Autodesk Inventor part; units mm, degrees
ref_plane "YZ Plane" through (0, 0, 0) normal (1, 0, 0) x (0, 1, 0)
ref_plane "XZ Plane" through (0, 0, 0) normal (0, 1, 0) x (-1, 0, 0)
ref_plane "XY Plane" through (0, 0, 0) normal (0, 0, 1) x (1, 0, 0)
sketch "Sketch1" plane through (0, 0, 0) normal (0, 1, 0) x (-1, 0, 0)
  line L0 (-21, -21) -> (21, -21)
  line L1 (21, -21) -> (21, 21)
  line L2 (21, 21) -> (-21, 21)
  line L3 (-21, 21) -> (-21, -21)
  line L4 (-21, -21) -> (21, 21) construction
  line L5 (21, -21) -> (-21, 21) construction
  point P0 (0, 0)
  dimension "d0" = 42
extrude "Extrusion1" add sketch "Sketch1" along normal blind 5
sketch "Sketch2" plane through (0, 0, 0) normal (0, 1, 0) x (1, 0, 0)
  circle A0 centre (0, 0) radius 21
  dimension "d3" = 42
extrude "Extrusion2" add sketch "Sketch2" along normal blind 51
sketch "Sketch3" plane through (0, 51, 0) normal (0, 1, 0) x (1, 0, 0)
  circle A0 centre (0, 0) radius 12.5
  dimension "d6" = 25
extrude "Extrusion3" add sketch "Sketch3" along normal blind 2
sketch "Sketch4" plane through (0, 51, 0) normal (0, 1, 0) x (1, 0, 0)
  circle A0 centre (0, 0) radius 4
  dimension "d9" = 8
extrude "Extrusion4" add sketch "Sketch4" along normal blind 22
sketch "Sketch5" plane through (0, 51, 0) normal (0, 1, 0) x (1, 0, 0)
  line L0 (-12.3744, -12.3744) -> (12.3744, -12.3744)
  line L1 (12.3744, -12.3744) -> (12.3744, 12.3744)
  line L2 (12.3744, 12.3744) -> (-12.3744, 12.3744)
  line L3 (-12.3744, 12.3744) -> (-12.3744, -12.3744)
  line L4 (-12.3744, -12.3744) -> (12.3744, 12.3744) construction
  line L5 (12.3744, -12.3744) -> (-12.3744, 12.3744) construction
  point P0 (0, 0)
  dimension "d15" = 35
hole "Hole1" at (12.3744, 51, -12.3744) at (-12.3744, 51, -12.3744) at (-12.3744, 51, 12.3744) at (12.3744, 51, 12.3744) direction (0, -1, 0) diameter 3.242 depth 6 tip angle 118
sketch "Sketch6" plane through (0, 73, 0) normal (0, 1, 0) x (1, 0, 0)
  point P0 (0, 0)
  point P1 (0, 0)
hole "Hole2" at (0, 73, 0) direction (0, -1, 0) diameter 2.459 depth 6 tip angle 118
chamfer "Chamfer1" distance 3 angle 45 4 edges at (21, 2.5, -21) (-21, 2.5, -21) (21, 2.5, 21) (-21, 2.5, 21)
sketch "Sketch7" plane through (0, 0, 0) normal (0, 1, 0) x (-1, 0, 0)
  circle A0 centre (0, 0) radius 11
  dimension "d30" = 22
extrude "Extrusion5" cut sketch "Sketch7" along normal blind 2
sketch "Sketch8" plane through (0, 0, 0) normal (0, 1, 0) x (-1, 0, 0)
  line L0 (15.5, 15.5) -> (-15.5, 15.5)
  line L1 (-15.5, 15.5) -> (-15.5, -15.5)
  line L2 (-15.5, -15.5) -> (15.5, -15.5)
  line L3 (15.5, -15.5) -> (15.5, 15.5)
  line L4 (15.5, 15.5) -> (-15.5, -15.5) construction
  line L5 (-15.5, 15.5) -> (15.5, -15.5) construction
  point P0 (0, 0)
  dimension "d33" = 31
hole "Hole3" at (15.5, 0, 15.5) at (-15.5, 0, 15.5) at (-15.5, 0, -15.5) at (15.5, 0, -15.5) direction (0, 1, 0) diameter 3.7 depth 5
sketch "Sketch9" plane through (0, 5, 0) normal (0, 1, 0) x (1, 0, 0)
  arc A0 (-15.9176, -13.6978) -> (-13.6978, -15.9176) centre (-15.5, -15.5) ccw
  circle A1 centre (-15.5, 15.5) radius 1.85
  arc A2 (15.9176, 13.6978) -> (13.6978, 15.9176) centre (15.5, 15.5) ccw
  circle A3 centre (15.5, -15.5) radius 1.85
  point P0 (0, 0)
hole "Hole4" at (-15.5, 5, 15.5) at (-15.5, 5, -15.5) at (15.5, 5, -15.5) at (15.5, 5, 15.5) direction (0, -1, 0) diameter 6.6 depth 3 tip angle 118
properties part number "911-42-reducer-long"
Work out the finished part from the listing and answer in its coordinate system (mm). A direction names the side the tool comes from. Coordinates: 2 decimals unless noted, no trailing zeros. Order: outer loops, then holes, each group sorted by start corner. A loop starts at its lowest first (then second) coordinate and runs counter-clockwise, first axis right, second up. Notation, with made-up numbers: (-14, 79.5) - (29, 79.5) arc R19 ccw to (29, 95.5) - close; hole circle Ø1 at (-29.5, 37). An arc over 180 degrees is marked (long way). Put each result on its own line as item: value. Start each with the question number.
1) Find section D-D (y = 34.5). Give the vertices of the cut face in (x, z).
2) Find section C-C (x = 6). Give the vertices of the cut face in (y, z), plus the area to 3 significant figures.
3) Find section B-B (z = -15.5). Give the vertices of the cut face in (x, y).
4) For faces 4 (the cylindrical face through (10.767, 47.958, 12.163)), 5 (the cylindrical face through (15.4, 3.5, -18.8)), 6 (the cylindrical face through (2.38, 0.99, 10.74)), 7 (the flat face through (18, 5, 18)), determine the directions among +Z, -Z, +X, -X, +Y, -Y from which every point of the face is accessible in a straight line to the end or side of a thin tool.
5) Find the intervals of material crossed by line 1 (Z direction, x = -15.5, y = 0.45); line 2 (X direction, y = 3, z = -15), in increasing order. Write a range as from..to.
6) For a pull along Y with two mould halves and no side action, classify faces 1 (the flat face through (-3, 53, -3)), 2 (the flat face through (-14, 5, -14)), 3 (the cylindrical face through (-10.792, 47.958, 12.023)) as released by +Y, released by -Y, zero draft, split by the parting line, or undercut.
7) Flat-ended cylindrical pins translate along their axes: pin 1 (3 mm diameter, centred on y = 9.5, z = 13, fed in from +X); pin 2 (1 mm diameter, centred on x = 2.5, y = 9, fed in from +Z); pin 3 (2.5 mm diameter, centred on x = 15, z = -15.5, fed in from -Y). Find the tip coordinate at first contact, or state that the pin passes through.
8) Find section A-A (x = -15.5). Give the vertices of the cut face in (y, z).
Results list:
1. outline: circle Ø42 at (0, 0)
2. outline: (0, -21) - (5, -21) - (5, -20.12) - (51, -20.12) - (51, -10.97) - (53, -10.97) - (53, 10.97) - (51, 10.97) - (51, 20.12) - (5, 20.12) - (5, 21) - (0, 21) - (0, 9.22) - (2, 9.22) - (2, -9.22) - (0, -9.22) - close
2. area: 2,070 mm^2
3. outline: (-21, 0) - (-17.35, 0) - (-17.35, 1.13) - (-18.8, 2) - (-18.8, 5) - (-21, 5) - close; (-14.17, 5) - (-12.2, 5) - (-12.2, 2) - (-13.65, 1.13) - (-13.65, 0) - (13.65, 0) - (13.65, 1.13) - (12.2, 2) - (12.2, 5) - (14.17, 5) - (14.17, 51) - (-14.17, 51) - close; (17.35, 0) - (21, 0) - (21, 5) - (18.8, 5) - (18.8, 2) - (17.35, 1.13) - close
4. face 4: +Y
4. face 5: none
4. face 6: -Y
4. face 7: +Z, +X, +Y
5. line 1: z = -21..-17.35, -13.65..13.65, 17.35..21
5. line 2: x = -21..-18.76, -12.24..12.24, 18.76..21
6. face 1: released by +Y
6. face 2: undercut
6. face 3: zero draft
7. pin 1: stops at x = 17.57
7. pin 2: stops at z = 20.9
7. pin 3: stops at y = 5
8. outline: (0, -21) - (5, -21) - (5, -18.8) - (2, -18.8) - (1.13, -17.35) - (0, -17.35) - close; (0, -13.65) - (1.13, -13.65) - (2, -12.2) - (5, -12.2) - (5, -14.17) - (51, -14.17) - (51, 14.17) - (5, 14.17) - (5, 12.2) - (2, 12.2) - (1.13, 13.65) - (0, 13.65) - close; (0, 17.35) - (1.13, 17.35) - (2, 18.8) - (5, 18.8) - (5, 21) - (0, 21) - close
